from build123d import *

# Parameters (mm, degrees)
SKETCH1_R           = 5.725
SKETCH1_R_2         = 3
BOSS_EXTRUDE1_DEPTH = 34
SKETCH2_R           = 5.725
BOSS_EXTRUDE2_DEPTH = 34
SKETCH3_R           = 2.6
CUT_EXTRUDE1_DEPTH  = 40
CUT_EXTRUDE2_DEPTH  = 4.7
SKETCH5_W           = 8.2
SKETCH5_H           = 4.7
CUT_EXTRUDE3_DEPTH  = 10
CUT_EXTRUDE10_DEPTH = 6


with BuildPart() as part:
    # Sketch1 → Boss-Extrude1 (new body)
    with BuildSketch(Plane(origin=(0, 0, 0), x_dir=(1, 0, 0), z_dir=(0, 1, 0))):
        with Locations(Location((0, 0, 0), (0, 0, 270))):
            Circle(SKETCH1_R)
        with Locations(Location((0, 0, 0), (0, 0, 270))):
            Circle(SKETCH1_R_2, mode=Mode.SUBTRACT)
    extrude(amount=BOSS_EXTRUDE1_DEPTH)

    # Sketch2 → Boss-Extrude2 (add)
    with BuildSketch(Plane(origin=(0, 0, 0), x_dir=(-1, 0, 0), z_dir=(0, -1, 0))):
        with Locations(Location((0, 0, 0), (0, 0, 270))):
            Circle(SKETCH2_R)
    extrude(amount=-BOSS_EXTRUDE2_DEPTH)

    # Sketch3 → Cut-Extrude1 (cut)
    with BuildSketch(Plane(origin=(0, 0, 0), x_dir=(-1, 0, 0), z_dir=(0, -1, 0))):
        with Locations(Location((0, 0, 0), (0, 0, 90))):
            Circle(SKETCH3_R)
    extrude(amount=-CUT_EXTRUDE1_DEPTH, mode=Mode.SUBTRACT)

    # Sketch4 → Cut-Extrude2 (cut)
    with BuildSketch(Plane(origin=(0, 7.2, 0), x_dir=(1, 0, 0), z_dir=(0, 1, 0))):
        Polygon((0, -4.734272207), (4.1, -2.367136104), (4.1, 2.367136104), (0, 4.734272207), (-4.1, 2.367136104), (-4.1, -2.367136104), align=None)
    extrude(amount=-CUT_EXTRUDE2_DEPTH, mode=Mode.SUBTRACT)

    # Sketch5 → Cut-Extrude3 (cut)
    with BuildSketch(Plane.XY):
        with Locations((0, 4.85)):
            Rectangle(SKETCH5_W, SKETCH5_H)
    extrude(amount=-CUT_EXTRUDE3_DEPTH, mode=Mode.SUBTRACT)

    # Sketch6 → Cut-Extrude10 (cut)
    with BuildSketch(Plane(origin=(0, 19.2, 0), x_dir=(1, 0, 0), z_dir=(0, 1, 0))):
        Polygon((-4.1, 2.367136104), (-4.1, -6.0044428), (-4.1, -15.659528102), (4.1, -15.659528102), (4.1, -2.367136104), (4.1, 2.367136104), align=None)
        Polygon((4.1, 2.367136104), (-4.1, 2.367136104), (0, 4.734272207), align=None)
    extrude(amount=CUT_EXTRUDE10_DEPTH, mode=Mode.SUBTRACT)


solid = part.part
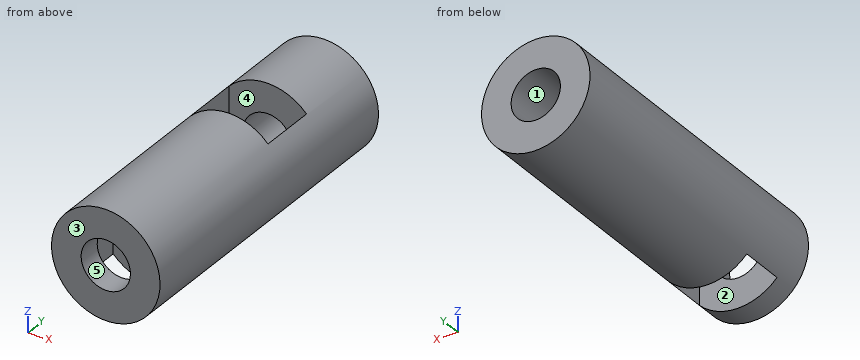
Check sheet for the modelled part. Datum: model origin and axes. Units: mm. Face numbers are marked on the shaded views. A direction names the side the tool comes from. Give positions to 0.01 mm unless a question says otherwise; leave off trailing zeros. Loops run counter-clockwise (first coordinate to the right, second up) from the corner with the lowest first, then second, coordinate; pieces in that order, holes last. Notation, with made-up numbers: M 46.25,54.25 L 51.25,54.25 A17 cw 51.25,61.25 Z; hole C 59.25,-23.75 d5. An arc over 180 degrees is marked long. Use a Markdown table: item, result. Add a question column.
Q1. Sectioned sample at B-B, the plane x = -3. Record the cut outline in (y, z), then the cut area to 3 significant figures.
Q2. Sectioned sample at C-C, the plane y = 13. Record the cut outline in (x, z) (3 decimals), then the cut area to 3 significant figures.
Q3. Sectioned sample at A-A, the plane z = 0. Record the cut outline in (x, y) (3 decimals).
Q4. Tool access check on the marked faces 4 and 5. Record the directions out of +Z, -Z, +X, -X, +Y, -Y that give a thin tool (end or side, any length) a straight path to the whole face; none if there is none.
Q5. Go/stop test with a flat-tipped pin: pin 1 (4 mm diameter, centred on y = 9.5, z = -3.5, fed in from -X) (3 decimals). Record where the tip stops, or that it passes through.
Q6. Sectioned sample at D-D, the plane z = -2. Record the cut outline in (x, y).
Q7. Mould release check, pull along Y, two halves, no side actions. Record for the marked faces 1, 2 and 3: pulls with the +Y half, pulls with the -Y half, needs draft (parallel to the pull), parting line crosses it, or undercut.
Q8. Scan lines: line 1 along Y through (x, z) = (3, -0.75); line 2 along X through (y, z) = (30, 0) (3 decimals); line 3 along Y through (x, z) = (3.5, -3.75). Record each from-to range of solid material in increasing order. Write a range as [from, to].
Verdict:
| question | item | result |
|---|---|---|
| 1 | outline | M 0,-4.88 L 2.5,-4.88 L 2.5,3 L 7.2,3 L 7.2,-4.88 L 34,-4.88 L 34,4.88 L 25.2,4.88 L 25.2,-3 L 19.2,-3 L 19.2,4.88 L 0,4.88 Z |
| 1 | area | 247 mm^2 |
| 2 | outline | C 0,0 d11.45; hole C 0,0 d5.2 |
| 2 | area | 81.7 mm^2 |
| 3 | outline | M -5.725,0 L -2.6,0 L -2.6,2.5 L -4.1,2.5 L -4.1,7.2 L -2.6,7.2 L -2.6,19.2 L -4.1,19.2 L -4.1,25.2 L -2.6,25.2 L -2.6,34 L -5.725,34 Z; M 2.6,0 L 5.725,0 L 5.725,34 L 2.6,34 L 2.6,25.2 L 4.1,25.2 L 4.1,19.2 L 2.6,19.2 L 2.6,7.2 L 4.1,7.2 L 4.1,2.5 L 2.6,2.5 Z |
| 4 | face 4 | +Z |
| 4 | face 5 | +Y, -Y |
| 5 | pin 1 | x = -5.525 |
| 6 | outline | M -5.36,0 L -1.66,0 L -1.66,2.5 L -4.1,2.5 L -4.1,7.2 L -1.66,7.2 L -1.66,19.2 L -4.1,19.2 L -4.1,25.2 L -1.66,25.2 L -1.66,34 L -5.36,34 Z; M 1.66,0 L 5.36,0 L 5.36,34 L 1.66,34 L 1.66,25.2 L 4.1,25.2 L 4.1,19.2 L 1.66,19.2 L 1.66,7.2 L 4.1,7.2 L 4.1,2.5 L 1.66,2.5 Z |
| 7 | face 1 | needs draft |
| 7 | face 2 | undercut |
| 7 | face 3 | pulls with the -Y half |
| 8 | line 1 | [0, 2.5], [7.2, 19.2], [25.2, 34] |
| 8 | line 2 | [-5.725, -2.6], [2.6, 5.725] |
| 8 | line 3 | [0, 2.5], [7.2, 34] |
